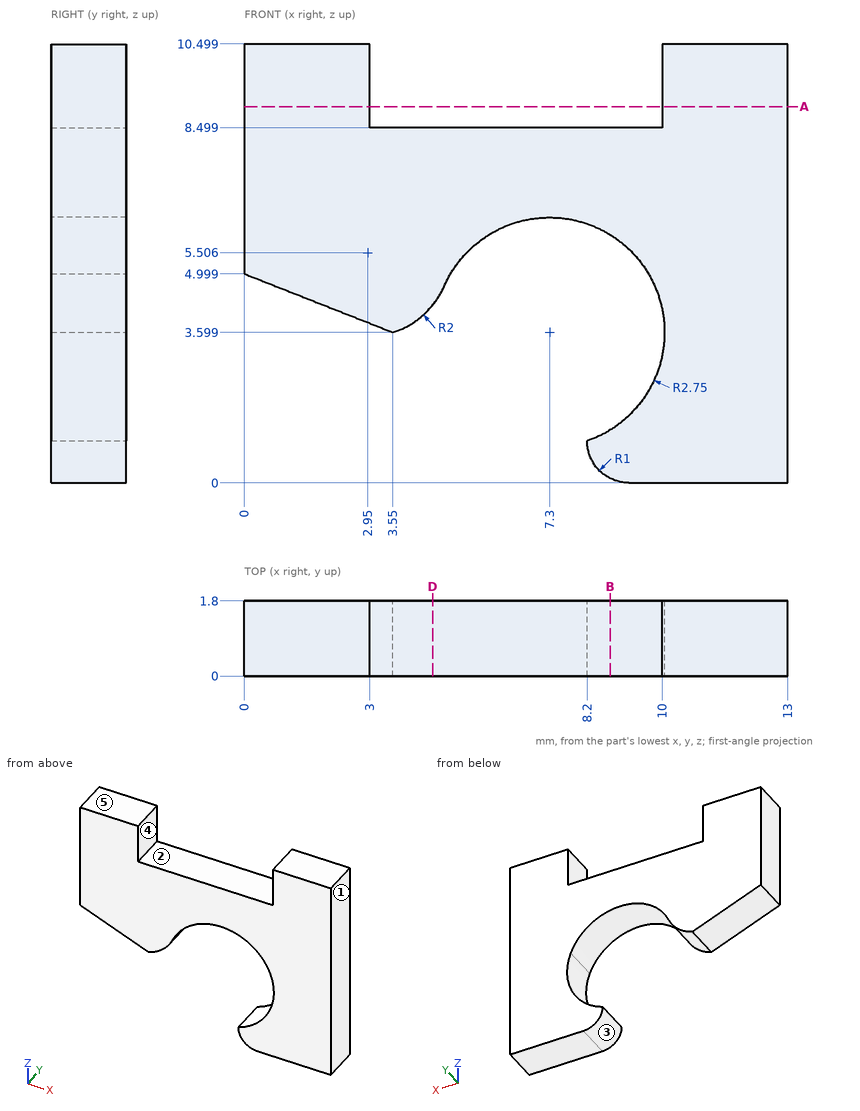
Design review of the part shown in the three views and the two pictorial views. Dimensions are in mm from the part's minimum x, y and z. A direction names the side the tool comes from. Round coordinates to 2 decimals unless told otherwise and drop trailing zeros. Order: outer loops, then holes, each group sorted by start corner. A loop starts at its lowest first (then second) coordinate and runs counter-clockwise, first axis right, second up.
(1) Take a section at B-B, the plane x = 8.75. State the section outline as (y, z) points (1 decimal).
Working result:
outline: (0, 0.1) - (1.8, 0.1) - (1.8, 1.3) - (0, 1.3) - close; (0, 5.9) - (1.8, 5.9) - (1.8, 8.5) - (0, 8.5) - close
(2) Take a section at A-A, the plane z = 9. State the section outline as (x, y) points.
Working result:
outline: (0, 0) - (3, 0) - (3, 1.8) - (0, 1.8) - close; (10, 0) - (13, 0) - (13, 1.8) - (10, 1.8) - close
(3) For P1, Ø0.5, axis at y = 0.5, z = 9, coming from the -X side, flat-tipped, find the tip position at first contact; note if it passes through.
Working result:
P1: stops at x = 0
(4) Take a section at D-D, the plane x = 4.5. State the section outline as (y, z) points.
Working result:
outline: (0, 4.24) - (1.8, 4.24) - (1.8, 8.5) - (0, 8.5) - close
(5) Wall thickness on L1, parallel to X at y = 0.55, z = 8.75; L2, parallel to X at y = 0.65, z = 3.5; L3, parallel to X at y = 1.5, z = 5.75 (1 decimal): over which ranges is each line inside the solid? List them lowest first.
Working result:
L1: x = 0 to 3, 10 to 13
L2: x = 10.05 to 13
L3: x = 0 to 5.6, 9 to 13
(6) Tool access review of the marked faces 1 and 2: name each direction out of +Z, -Z, +X, -X, +Y, -Y from which nothing blocks a thin tool from reaching the whole face with its end or side.
Working result:
face 1: +Z, -Z, +X, +Y, -Y
face 2: +Z, +Y, -Y
(7) Mouldability with a two-part tool opening along X and no side actions: class the marked faces 3, 4 and 5 as released by +X, released by -X, zero draft, split by the parting line, or undercut.
Working result:
face 3: released by -X
face 4: undercut
face 5: zero draft
